Input: dimensioned drawing with shaded views. Units: mm. Origin: part minimum x, y, z. Give positions to 0.01 mm unless a question says otherwise; leave off trailing zeros. Loops run counter-clockwise (first coordinate to the right, second up) from the corner with the lowest first, then second, coordinate; pieces in that order, holes last. Notation, with made-up numbers: (22, -27.75) -> (37, -27.75) arc R36 ccw to (37, 7.25) -> close; hole circle Ø8 at (42, -20). An arc over 180 degrees is marked (long way). Answer in a Markdown table with one row per item. Add a question column.
1) Section query B-B (y = 22). Return the cut outline in (x, z) (1 decimal), plus the area to 3 significant figures.
2) Draft query along Z for the marked faces 1, 2 and 3. Return one class per face: +Z half, -Z half, draft (parallel to the pull), parting line (faces both ways), or undercut.
3) Line query: line 1 (X direction, y = 40, z = 19) (1 decimal); line 2 (Z direction, x = 19.05, y = 55.5) (1 decimal); line 3 (Z direction, x = 209.5, y = 59) (1 decimal). Output: solid intervals per line, ascending. Write a range as from..to.
4) First-contact query: P1, Ø8, axis at x = 48, y = 20.5, coming from the +Z side; P2, Ø2, axis at x = 26.5, y = 25, coming from the +Z side; P3, Ø4, axis at y = 17, z = 163, coming from the -X side; P4, Ø1, axis at x = 113.5, z = 185, coming from the -Y side. Flat tips, straight axial feed; report the tip coordinate or a pass-through.
5) Section query A-A (z = 248.92). Return the cut outline in (x, y) (1 decimal), plus the area to 3 significant figures.
6) Section query C-C (z = 164). Give the number of separate pieces and of enclosed holes in the cut face.
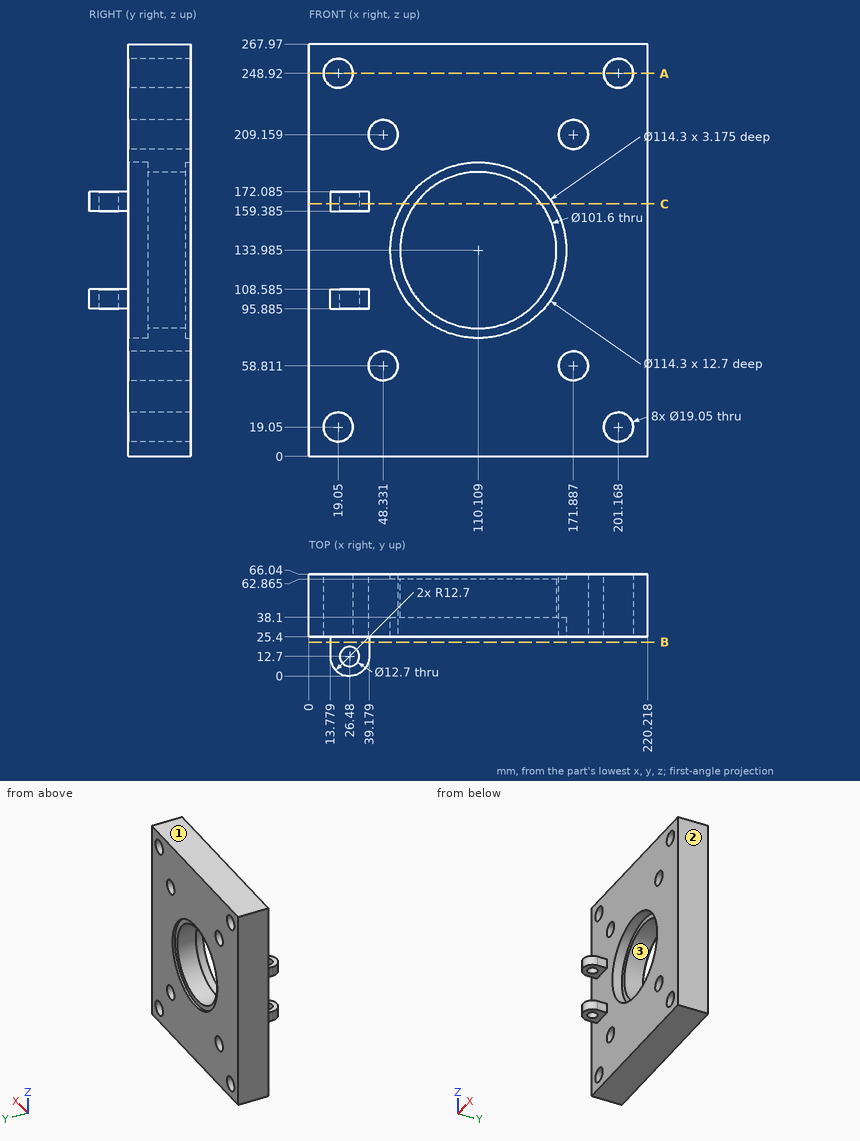
Evaluation:
| question | item | result |
|---|---|---|
| 1 | outline | (13.8, 95.9) -> (39.2, 95.9) -> (39.2, 108.6) -> (13.8, 108.6) -> close; (13.8, 159.4) -> (39.2, 159.4) -> (39.2, 172.1) -> (13.8, 172.1) -> close |
| 1 | area | 645 mm² |
| 2 | face 1 | +Z half |
| 2 | face 2 | draft |
| 2 | face 3 | undercut |
| 3 | line 1 | 0..9.5, 28.6..191.6, 210.7..220.2 |
| 3 | line 2 | 0..9.5, 28.6..239.4, 258.4..268 |
| 3 | line 3 | 0..14.4, 23.7..244.3, 253.5..268 |
| 4 | P1 | through |
| 4 | P2 | z = 267.97 |
| 4 | P3 | x = 13.78 |
| 4 | P4 | y = 38.1 |
| 5 | outline | (0, 25.4) -> (9.5, 25.4) -> (9.5, 66) -> (0, 66) -> close; (28.6, 25.4) -> (191.6, 25.4) -> (191.6, 66) -> (28.6, 66) -> close; (210.7, 25.4) -> (220.2, 25.4) -> (220.2, 66) -> (210.7, 66) -> close |
| 5 | area | 7,400 mm² |
| 6 | separate pieces | 2 |
| 6 | enclosed holes | 1 |
